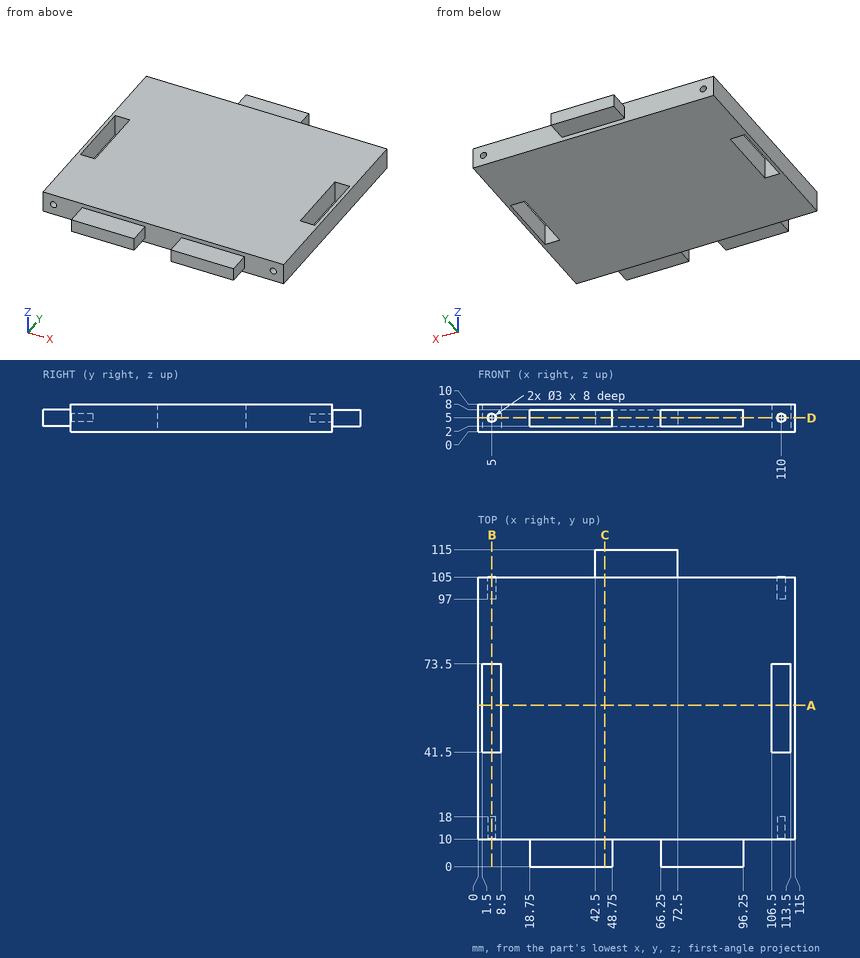
Answer from the drawing. Dimensions are ordinates in mm from the lowest x, y and z of the part. Give positions to 0.01 mm unless a question says otherwise; leave off trailing zeros. Loops run counter-clockwise (first coordinate to the right, second up) from the corner with the lowest first, then second, coordinate; pieces in that order, holes last. Notation, with made-up numbers: (71.5, 38.25) -> (101.5, 38.25) arc R29 cw to (101.5, 73.25) -> close; hole circle Ø5 at (-19.75, 57). An arc over 180 degrees is marked (long way). Answer as CSV lines item,"result".
Item 1: Each of these flat-tipped pins is pushed along its axis until it touches: pin 1 (1.5 mm diameter, centred on x = 12.5, z = 1, fed in from -Y); pin 2 (5.5 mm diameter, centred on x = 3.5, z = 5, fed in from +Y); pin 3 (2.5 mm diameter, centred on x = 110, z = 5, fed in from +Y). Where does it stop, or does it pass through?
Returned:
pin 1,"stops at y = 10"
pin 2,"stops at y = 105"
pin 3,"stops at y = 97"
Item 2: Find section B-B on x = 5. Give the vertices of the cut face in (y, z).
Returned:
outline,"(10, 0) -> (41.5, 0) -> (41.5, 10) -> (10, 10) -> (10, 6.5) -> (18, 6.5) -> (18, 3.5) -> (10, 3.5) -> close; (73.5, 0) -> (105, 0) -> (105, 3.5) -> (97, 3.5) -> (97, 6.5) -> (105, 6.5) -> (105, 10) -> (73.5, 10) -> close"
Item 3: Find section D-D on z = 5. State how many separate pieces and enclosed holes the cut face has, plus the area to 3 significant figures.
Returned:
separate pieces,"1"
enclosed holes,"2"
area,"11,300 mm²"
Item 4: Find section C-C on x = 46. Give the vertices of the cut face in (y, z).
Returned:
outline,"(0, 2) -> (10, 2) -> (10, 0) -> (105, 0) -> (105, 2) -> (115, 2) -> (115, 8) -> (105, 8) -> (105, 10) -> (10, 10) -> (10, 8) -> (0, 8) -> close"
Item 5: Consider line 1 (X direction, y = 57, z = 7.25); line 2 (Z direction, x = 110, y = 102); line 3 (X direction, y = 103.25, z = 5). Determine where each line is inside the solid, lowest interval first. Write a range as [from, to].
Returned:
line 1,"x = [0, 1.5], [8.5, 106.5], [113.5, 115]"
line 2,"z = [0, 3.5], [6.5, 10]"
line 3,"x = [0, 3.5], [6.5, 108.5], [111.5, 115]"
Item 6: Find section A-A on y = 58.5. Give the vertices of the cut face in (x, z), plus the area to 3 significant figures.
Returned:
outline,"(0, 0) -> (1.5, 0) -> (1.5, 10) -> (0, 10) -> close; (8.5, 0) -> (106.5, 0) -> (106.5, 10) -> (8.5, 10) -> close; (113.5, 0) -> (115, 0) -> (115, 10) -> (113.5, 10) -> close"
area,"1,010 mm²"
